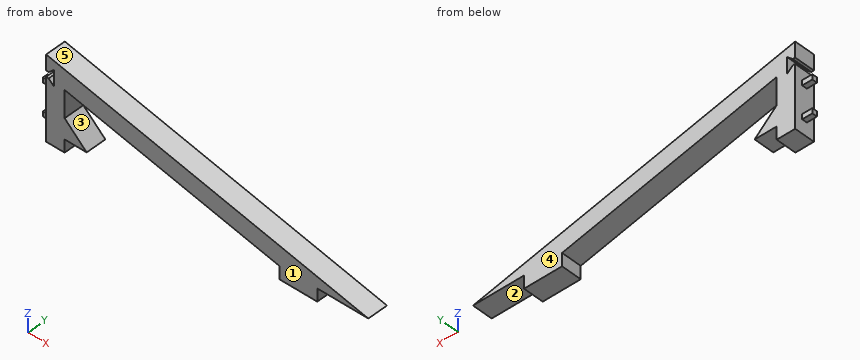
```python
from build123d import *

# Parameters (mm, degrees)
P_IDAT_VYSUNUT_M1_DEPTH  = 8
ODEBRAT_VYSUNUT_M1_DEPTH = 132.589517946
SKICA3_W                 = 2
SKICA3_H                 = 2
P_IDAT_VYSUNUT_M2_DEPTH  = 4
SKICA5_W                 = 16
SKICA5_H                 = 8
P_IDAT_VYSUNUT_M4_DEPTH  = 8
ODEBRAT_VYSUNUT_M3_DEPTH = 132.589517946


with BuildPart() as part:
    # Skica1 → Přidat vysunutím1 (new body)
    with BuildSketch(Plane(origin=(0, 0, 0), x_dir=(1, 0, 0), z_dir=(0, 1, 0))):
        Polygon((0, 0), (0, -32.97), (127.140789416, -5), (107, -5), (107, 0), (92, 0), (92, -5.051361455), (7.3, -23.684712804), (7.3, 0), align=None)
    extrude(amount=P_IDAT_VYSUNUT_M1_DEPTH)

    # Skica2 → Odebrat vysunutím1 (cut, through all)
    with BuildSketch(Plane(origin=(0, 8, 0), x_dir=(1, 0, 0), z_dir=(0, 1, 0))):
        Polygon((0, -24.5), (1, -24.5), (3.2, -22.5), (3.2, -28.9), (1, -26.9), (0, -26.9), align=None)
    extrude(amount=-ODEBRAT_VYSUNUT_M1_DEPTH, mode=Mode.SUBTRACT)

    # Skica3 → Přidat vysunutím2 (add)
    with BuildSketch(Plane.ZY):
        with Locations((6.4, 4)):
            Rectangle(SKICA3_W, SKICA3_H)
        with Locations((19.2, 4)):
            Rectangle(SKICA3_W, SKICA3_H)
    extrude(amount=P_IDAT_VYSUNUT_M2_DEPTH)

    # Skica5 → Přidat vysunutím4 (add)
    with BuildSketch(Plane(origin=(0, 8, 0), x_dir=(1, 0, 0), z_dir=(0, 1, 0))):
        with Locations((8, -9)):
            Rectangle(SKICA5_W, SKICA5_H)
    extrude(amount=-P_IDAT_VYSUNUT_M4_DEPTH)

    # Skica7 → Odebrat vysunutím3 (cut, through all)
    with BuildSketch(Plane.XZ):
        Polygon((7.3, 13), (16, 13), (16, 5), align=None)
    extrude(amount=-ODEBRAT_VYSUNUT_M3_DEPTH, mode=Mode.SUBTRACT)


solid = part.part
```
Can you work these out from the model? Positions are in its coordinate system, mm. Face numbers are marked on the shaded views. A direction names the side the tool comes from. Coordinates: 2 decimals unless noted, no trailing zeros. Loops run counter-clockwise (first coordinate to the right, second up) from the corner with the lowest first, then second, coordinate; pieces in that order, holes last.
1) Imagine slicing it at A-A on z = 2.5. List the corners of the cut face in (x, y) for me, plus the area to 3 significant figures.
2) Imagine slicing it at D-D on x = 119. List the corners of the cut face in (y, z) for me.
3) Thinking about a two-plate mould opening in X: for the marked faces 3, 4 and 5, which applies, pulls with the +X half, pulls with the -X half, needs draft (parallel to the pull), parting line crosses it, or undercut?
4) Imagine slicing it at C-C on y = 6.25. List the corners of the cut face in (x, z) for me, plus the area to 3 significant figures.
5) Imagine slicing it at B-B on x = 9. List the corners of the cut face in (y, z) for me, plus the area to 3 significant figures.
6) Which directions (+Z, -Z, +X, -X, +Y, -Y) give clear straight access to the entire face, cutting with the end or side of a thin tool? Please do the marked faces 1 and 2.
7) For pin 1 (2 mm diameter, centred on x = 22, y = 3, fed in from +Z); pin 2 (2 mm diameter, centred on x = -2.5, y = 4.5, fed in from +Z); pin 3 (3 mm diameter, centred on x = 43, y = 2.5, fed in from -Z), each with a flat end and sliding along its axis, tell me the tip position at first contact or that it passes through.
8) I need wall thicknesses on probe 1 along X at (y, z) = (3.5, 3); probe 2 along Z at (x, y) = (9.5, 0.5); probe 3 along Z at (x, y) = (79.5, 4). Which ranges of each line are inside material? Lowest first, please.
Completed:
1. outline: (0, 0) - (7.3, 0) - (7.3, 8) - (0, 8) - close; (92, 0) - (107, 0) - (107, 8) - (92, 8) - close
1. area: 178 mm2
2. outline: (0, 5) - (8, 5) - (8, 6.79) - (0, 6.79) - close
3. face 3: undercut
3. face 4: needs draft
3. face 5: pulls with the +X half
4. outline: (0, 0) - (7.3, 0) - (7.3, 5) - (16, 5) - (7.3, 13) - (7.3, 23.68) - (92, 5.05) - (92, 0) - (107, 0) - (107, 5) - (127.14, 5) - (0, 32.97) - (0, 26.9) - (1, 26.9) - (3.2, 28.9) - (3.2, 22.5) - (1, 24.5) - (0, 24.5) - close
4. area: 1,120 mm2
5. outline: (0, 5) - (8, 5) - (8, 11.44) - (0, 11.44) - close; (0, 23.31) - (8, 23.31) - (8, 30.99) - (0, 30.99) - close
5. area: 113 mm2
6. face 1: +Z, -Z, +X, -X, -Y
6. face 2: -Z, +X, +Y, -Y
7. pin 1: stops at z = 28.35
7. pin 2: stops at z = 20.2
7. pin 3: stops at z = 15.5
8. probe 1: x = 0 to 7.3, 92 to 107
8. probe 2: z = 5 to 10.98, 23.2 to 30.88
8. probe 3: z = 7.8 to 15.48
